Geometry check sheet. Reference: the model listing, model coordinates, mm. A direction names the side the tool comes from. Coordinates: 2 decimals unless noted, no trailing zeros. Loops run counter-clockwise (first coordinate to the right, second up) from the corner with the lowest first, then second, coordinate; pieces in that order, holes last. Notation, with made-up numbers: (-7.75, -33.75) -> (9.25, -33.75) arc R22 cw to (9.25, -26.75) -> close; hole circle Ø6 at (19.25, 83.25). An arc over 180 degrees is marked (long way). Answer as a JSON object with one key per item and string values.
from build123d import *

# Parameters (mm, degrees)
SKETCH1_R           = 4
BOSS_EXTRUDE1_DEPTH = 35
SKETCH2_W           = 8
SKETCH2_H           = 2.52995071
CUT_EXTRUDE1_DEPTH  = 10


with BuildPart() as part:
    # Sketch1 → Boss-Extrude1 (new body, symmetric)
    with BuildSketch(Plane.XY):
        Circle(SKETCH1_R)
    extrude(amount=BOSS_EXTRUDE1_DEPTH, both=True)

    # Sketch2 → Cut-Extrude1 (cut)
    with BuildSketch(Plane.XY.offset(35)):
        Polygon((-4, -2), (4, -2), (4, -4.561964496), (-4, -4.711362164), align=None)
        with Locations((0, 3.264975355)):
            Rectangle(SKETCH2_W, SKETCH2_H)
    extrude(amount=-CUT_EXTRUDE1_DEPTH, mode=Mode.SUBTRACT)


solid = part.part
1. Thickness scan on probe 1 along X at (y, z) = (-2, 22); probe 2 along Y at (x, z) = (-0.25, -11). Record the ranges inside material, lowest first. Write a range as from..to.
Evaluation:
{"probe 1": "x = -3.46..3.46", "probe 2": "y = -3.99..3.99"}
2. Section check B-B, the plane z = -28.5. Record the boundary of the cut face in (x, y).
Evaluation:
{"outline": "circle Ø8 at (0, 0)"}
3. Section check D-D, the plane y = -1.25. Record the boundary of the cut face in (x, z).
Evaluation:
{"outline": "(-3.8, -35) -> (3.8, -35) -> (3.8, 35) -> (-3.8, 35) -> close"}
4. Tool access check on faces 1 (the face through (0, -2, 30)), 2 (the face through (0, 3, 25)), 3 (the face through (3.695, -1.532, 0.49)). Record the directions out of +Z, -Z, +X, -X, +Y, -Y that give a thin tool (end or side, any length) a straight path to the whole face; none if there is none.
Evaluation:
{"face 1": "+Z, +X, -X, -Y", "face 2": "+Z, +X, -X, +Y", "face 3": "+Z, -Z"}
5. Section check C-C, the plane x = 2.5. Record the boundary of the cut face in (y, z), then the cut area to 3 significant figures.
Evaluation:
{"outline": "(-3.12, -35) -> (3.12, -35) -> (3.12, 25) -> (2, 25) -> (2, 35) -> (-2, 35) -> (-2, 25) -> (-3.12, 25) -> close", "area": "415 mm^2"}
6. Depth check by flat-ended pin: P1, Ø2, axis at x = 1.5, z = 30, coming from the +Y side; P2, Ø2, axis at x = 0.5, z = 32, coming from the -Y side; P3, Ø1, axis at x = 0, y = 3.5, coming from the +Z side. Enter the tip coordinate at first touch or a pass-through.
Evaluation:
{"P1": "stops at y = 2", "P2": "stops at y = -2", "P3": "stops at z = 25"}
7. Section check A-A, the plane x = 0. Record the boundary of the cut face in (y, z).
Evaluation:
{"outline": "(-4, -35) -> (4, -35) -> (4, 25) -> (2, 25) -> (2, 35) -> (-2, 35) -> (-2, 25) -> (-4, 25) -> close"}
